```python
from build123d import *

# Parameters (mm, degrees)
EXTRUDE_2_DEPTH                = 5
SKETCH_4_W                     = 8.676470589
SKETCH_4_H                     = 35
SKETCH_4_W_2                   = 8.676470588
EXTRUDE_15_DEPTH               = 35
CUT_EXTRUDE_1_DEPTH            = 45
SKETCH_6_R                     = 14
CUT_EXTRUDE_2_DEPTH            = 45
FILLET_1_R                     = 5
SKETCH_7_R                     = 15
SKETCH_7_R_2                   = 13
EXTRUDE_16_DEPTH               = 1
SPLIT_BODIES_1_SURFACE_1_BACK  = 86
SPLIT_BODIES_1_SURFACE_1_DEPTH = 172
SPLIT_BODIES_1_SURFACE_2_BACK  = 86
SPLIT_BODIES_1_SURFACE_2_DEPTH = 172
SKETCH_17_W                    = 3
SKETCH_17_H                    = 13
EXTRUDE_20_DEPTH               = 42
EXTRUDE_21_DEPTH               = 3
SKETCH_19_R                    = 1.6
CUT_EXTRUDE_3_DEPTH            = 3
EXTRUDE_22_DEPTH               = 5
EXTRUDE_START                  = -3
EXTRUDE_25_DEPTH               = 3
HOLE_WIZARD_1_D                = 4.3
HOLE_WIZARD_1_DEPTH            = 5
HOLE_WIZARD_1_CBORE_D          = 10
HOLE_WIZARD_1_CBORE_DEPTH      = 0.5
HOLE_WIZARD_1_TIP              = 1.291850331
FILLET_2_R                     = 6


with BuildPart() as part:
    # 草图2 → 凸台-拉伸2 (new body)
    with BuildSketch(Plane.XY):
        Polygon((7.726423565, 24.338235294), (-14.773576435, 24.338235294), (-14.773576435, -35.661764706), (7.726423565, -35.661764706), (7.726423565, -23.161764706), (-6.097105846, -23.161764706), (-6.097105846, 11.838235294), (7.726423565, 11.838235294), align=None)
        Polygon((30.226423565, 24.338235294), (7.726423565, 24.338235294), (7.726423565, 11.838235294), (21.549952977, 11.838235294), (21.549952977, -23.161764706), (7.726423565, -23.161764706), (7.726423565, -35.661764706), (30.226423565, -35.661764706), align=None)
    extrude(amount=EXTRUDE_2_DEPTH)

    # 草图4 → 凸台-拉伸15 (add)
    with BuildSketch(Plane.XY.offset(5)):
        with Locations((-10.435341141, -5.661764706)):
            Rectangle(SKETCH_4_W, SKETCH_4_H)
        with Locations((25.888188271, -5.661764706)):
            Rectangle(SKETCH_4_W_2, SKETCH_4_H)
    extrude(amount=EXTRUDE_15_DEPTH)

    # 草图5 → 切除-拉伸1 (cut)
    with BuildSketch(Plane.ZY.offset(14.773576435)):
        with BuildLine():
            Line((40, -23.161764706), (40, -5.661764706))
            ThreePointArc((40, -5.661764706), (34.874368671, -18.036133377), (22.5, -23.161764706))
            Line((22.5, -23.161764706), (40, -23.161764706))
        make_face()
        with BuildLine():
            ThreePointArc((22.5, 11.838235294), (34.874368671, 6.712603965), (40, -5.661764706))
            Line((40, -5.661764706), (40, 11.838235294))
            Line((40, 11.838235294), (22.5, 11.838235294))
        make_face()
    extrude(amount=-CUT_EXTRUDE_1_DEPTH, mode=Mode.SUBTRACT)

    # 草图6 → 切除-拉伸2 (cut)
    with BuildSketch(Plane.ZY.offset(14.773576435)):
        with Locations((22.5, -5.661764706)):
            Circle(SKETCH_6_R)
    extrude(amount=-CUT_EXTRUDE_2_DEPTH, mode=Mode.SUBTRACT)

    # 圆角1
    fillet_1_edges = [part.edges().sort_by_distance(p)[0] for p in [
        (-6.097105846, 11.838235294, 2.5),
        (-6.097105846, -23.161764706, 2.5),
        (21.549952977, -23.161764706, 2.5),
        (21.549952977, 11.838235294, 2.5),
    ]]
    fillet(fillet_1_edges, radius=FILLET_1_R)

    # 草图7 → 凸台-拉伸16 (add)
    with BuildSketch(Plane(origin=(-6.097105846, 0, 0), x_dir=(0, 0, -1), z_dir=(1, 0, 0))):
        with Locations((-22.5, -5.661764706)):
            Circle(SKETCH_7_R)
        with Locations((-22.5, -5.661764706)):
            Circle(SKETCH_7_R_2, mode=Mode.SUBTRACT)
    extrude(amount=-EXTRUDE_16_DEPTH)


with BuildPart() as body_2:
    # Split Bodies 1: the piece behind the surface
    add(part.part)
    # Split Bodies 1 surface: a surface, the sketch's curves swept straight by 172 mm
    with BuildLine(Plane.XY.offset(5).offset(-SPLIT_BODIES_1_SURFACE_1_BACK), mode=Mode.PRIVATE) as split_bodies_1_surface_1_path:
        Line((7.726423565, 24.338235294), (7.726423565, -35.661764706))
    split_bodies_1_surface_1 = Shell.extrude(split_bodies_1_surface_1_path.wire(), (0 * SPLIT_BODIES_1_SURFACE_1_DEPTH, 0 * SPLIT_BODIES_1_SURFACE_1_DEPTH, 1 * SPLIT_BODIES_1_SURFACE_1_DEPTH))
    split(bisect_by=split_bodies_1_surface_1, keep=Keep.BOTTOM)


with BuildPart() as part_1:
    add(part.part)

    # Split Bodies 1: split by a surface, the side it looks to stays
    # Split Bodies 1 surface: a surface, the sketch's curves swept straight by 172 mm
    with BuildLine(Plane.XY.offset(5).offset(-SPLIT_BODIES_1_SURFACE_2_BACK), mode=Mode.PRIVATE) as split_bodies_1_surface_2_path:
        Line((7.726423565, 24.338235294), (7.726423565, -35.661764706))
    split_bodies_1_surface_2 = Shell.extrude(split_bodies_1_surface_2_path.wire(), (0 * SPLIT_BODIES_1_SURFACE_2_DEPTH, 0 * SPLIT_BODIES_1_SURFACE_2_DEPTH, 1 * SPLIT_BODIES_1_SURFACE_2_DEPTH))
    split(bisect_by=split_bodies_1_surface_2, keep=Keep.TOP)

    # 草图17 → 凸台-拉伸20 (add)
    with BuildSketch(Plane.XY.offset(5)):
        with Locations((28.726423565, -36.661764706)):
            Rectangle(SKETCH_17_W, SKETCH_17_H)
        with Locations((28.726423565, 23.338235294)):
            Rectangle(SKETCH_17_W, SKETCH_17_H)
    extrude(amount=EXTRUDE_20_DEPTH)

    # 草图18 → 凸台-拉伸21 (add)
    with BuildSketch(Plane(origin=(30.226423565, 0, 0), x_dir=(0, 0, -1), z_dir=(1, 0, 0))):
        with BuildLine():
            Line((-47, -30.161764706), (-47, -43.161764706))
            ThreePointArc((-47, -43.161764706), (-53.5, -36.661764706), (-47, -30.161764706))
        make_face()
        with BuildLine():
            Line((-47, 16.838235294), (-47, 29.838235294))
            ThreePointArc((-47, 29.838235294), (-53.5, 23.338235294), (-47, 16.838235294))
        make_face()
    extrude(amount=-EXTRUDE_21_DEPTH)

    # 草图19 → 切除-拉伸3 (cut)
    with BuildSketch(Plane(origin=(30.226423565, 0, 0), x_dir=(0, 0, -1), z_dir=(1, 0, 0))):
        with Locations((-47, 23.338235294)):
            Circle(SKETCH_19_R)
        with Locations((-47, -36.661764706)):
            Circle(SKETCH_19_R)
        with Locations((-10, 23.338235294)):
            Circle(SKETCH_19_R)
        with Locations((-10, -36.661764706)):
            Circle(SKETCH_19_R)
    extrude(amount=-CUT_EXTRUDE_3_DEPTH, mode=Mode.SUBTRACT)

    # 草图21 → 凸台-拉伸22 (add)
    with BuildSketch(Plane.XY.offset(5)):
        Polygon((18.226423565, -35.661764706), (30.226423565, -35.661764706), (30.226423565, -43.161764706), (27.226423565, -43.161764706), (26.408241747, -43.161764706), align=None)
        Polygon((18.226423565, 24.338235294), (30.226423565, 24.338235294), (30.226423565, 29.838235294), (26.476423565, 29.838235294), align=None)
    extrude(amount=-EXTRUDE_22_DEPTH)

    # 草图24 → 凸台-拉伸25 (add)
    with BuildSketch(Plane(origin=(30.226423565, 0, 0), x_dir=(0, 0, -1), z_dir=(1, 0, 0)).offset(EXTRUDE_START)):
        with BuildLine():
            Line((-5, 16.838235294), (-38, 16.838235294))
            ThreePointArc((-38, 16.838235294), (-36.230441453, 9.650254496), (-38, 2.462273699))
            ThreePointArc((-38, 2.462273699), (-31.557574949, 9.311890026), (-22.5, 11.838235294))
            Line((-22.5, 11.838235294), (-5, 11.838235294))
            Line((-5, 11.838235294), (-5, 16.838235294))
        make_face()
        with BuildLine():
            Line((-5, -30.161764706), (-38, -30.161764706))
            ThreePointArc((-38, -30.161764706), (-35.984258471, -21.973783908), (-38, -13.785803111))
            ThreePointArc((-38, -13.785803111), (-31.557574949, -20.635419438), (-22.5, -23.161764706))
            Line((-22.5, -23.161764706), (-5, -23.161764706))
            Line((-5, -23.161764706), (-5, -30.161764706))
        make_face()
    extrude(amount=EXTRUDE_25_DEPTH)

    # 打孔尺寸(%根据六角头螺)栓 全螺纹的类型1
    with Locations(Plane(origin=(18.226423565, 18.088235294, 5), x_dir=(1, 0, 0), z_dir=(0, 0, 1))):
        with Locations((0, 0), (0, -47.5)):
            CounterBoreHole(HOLE_WIZARD_1_D / 2, HOLE_WIZARD_1_CBORE_D / 2, HOLE_WIZARD_1_CBORE_DEPTH, depth=HOLE_WIZARD_1_DEPTH)
            with Locations((0, 0, -(HOLE_WIZARD_1_DEPTH + HOLE_WIZARD_1_TIP / 2))):  # 118° drill point
                Cone(0, HOLE_WIZARD_1_D / 2, HOLE_WIZARD_1_TIP, mode=Mode.SUBTRACT)

    # 圆角2
    fillet_2_edges = [part_1.edges().sort_by_distance(p)[0] for p in [
        (18.226423565, -35.661764706, 2.5),
        (18.226423565, 24.338235294, 2.5),
    ]]
    fillet(fillet_2_edges, radius=FILLET_2_R)


solid = part_1.part
```
Part model, mm, in its own coordinate system. A direction names the side the tool comes from. Coordinates: 2 decimals unless noted, no trailing zeros. Order: outer loops, then holes, each group sorted by start corner. A loop starts at its lowest first (then second) coordinate and runs counter-clockwise, first axis right, second up. Notation, with made-up numbers: (-9.75, 48.25) - (2.25, 48.25) arc R25 ccw to (2.25, 77.25) - close; hole circle Ø11 at (71.25, 42). An arc over 180 degrees is marked (long way). Return JSON: item names as keys, results as strings. Group by question number.
Item 1: Which spindle directions (+Z, -Z, +X, -X, +Y, -Y) get a long thin tool onto all of the face, cutting with end or side? Do faces 4 (the face through (24, 11.838, 14)), 5 (the face through (29, -30.162, 42)), 6 (the face through (12, -23.162, 2)), 7 (the face through (12, 24.338, 2)), 8 (the face through (27.226, -35, 29)). Say none if no direction does.
Item 2: Cut at A-A (z = 16). List the corners of the cut face in (x, y).
Item 3: Pin check, flat tips, straight feed: pin 1 (5 mm diameter, centred on x = 20, y = -29.5, fed in from +Z); pin 2 (10 mm diameter, centred on x = 16.5, z = 5.5, fed in from -Y); pin 3 (10 mm diameter, centred on x = 14, y = -26.5, fed in from +Z). Stop position of each tip, or through.
Item 4: Pull direction Z, two halves, no side cores. Call faces 1 (the face through (7.726, 18, 2)), 2 (the face through (24, -6, 0)), 3 (the face through (28.7, -38.1, 46.3)): pulls with the +Z half, pulls with the -Z half, needs draft (parallel to the pull), parting line crosses it, or undercut.
Item 5: Cut at B-B (z = 10). List the corners of the cut face in (x, y), plus the area to 3 significant figures.
Item 6: Cut at C-C (x = 28.75). List the corners of the cut face in (y, z).
Item 7: Cut at D-D (z = 30.5). List the corners of the cut face in (x, y).
Item 8: Drill centre lines: probe 1 along Y at (x, z) = (28.85, 10); probe 2 along Z at (x, y) = (23.25, 17); probe 3 along X at (y, z) = (-30, 10.5). Where is each one in solid material? Low to high. Write a range as from..to.
Check values:
{
 "1": {"face 4": "+Z, -X, +Y", "face 5": "+Z, +X, -X", "face 6": "+Z, -Z, -X", "face 7": "+Z, -Z, -X, +Y", "face 8": "+Z, -X, -Y"},
 "2": {"outline": "(21.55, -23.16) - (27.23, -23.16) - (27.23, -43.16) - (30.23, -43.16) - (30.23, -18.06) - (21.55, -18.06) - close; (21.55, 6.74) - (30.23, 6.74) - (30.23, 29.84) - (27.23, 29.84) - (27.23, 11.84) - (21.55, 11.84) - close"},
 "3": {"pin 1": "stops at z = 4.5", "pin 2": "stops at y = -38.64", "pin 3": "stops at z = 5"},
 "4": {"face 1": "needs draft", "face 2": "pulls with the -Z half", "face 3": "undercut"},
 "5": {"outline": "(21.55, -23.16) - (27.23, -23.16) - (27.23, -35.06) - (30.23, -35.06) - (30.23, -11.97) - (21.55, -11.97) - close; (21.55, 0.64) - (30.23, 0.64) - (30.23, 21.74) - (27.23, 21.74) - (27.23, 11.84) - (21.55, 11.84) - close; (27.23, -43.16) - (30.23, -43.16) - (30.23, -38.26) - (27.23, -38.26) - close; (27.23, 24.94) - (30.23, 24.94) - (30.23, 29.84) - (27.23, 29.84) - close", "area": "289 mm2"},
 "6": {"outline": "(-43.16, 0) - (29.84, 0) - (29.84, 47) arc R6.5 ccw to (16.84, 47) - (16.84, 38) arc R15.48 cw to (2.46, 38) arc R17.5 ccw to (-13.79, 38) arc R17.64 cw to (-30.16, 38) - (-30.16, 47) arc R6.5 ccw to (-43.16, 47) - close; hole circle Ø3.2 at (-36.66, 10); hole circle Ø3.2 at (-36.66, 47); hole circle Ø28 at (-5.66, 22.5); hole circle Ø3.2 at (23.34, 10); hole circle Ø3.2 at (23.34, 47)"},
 "7": {"outline": "(21.55, -21.23) - (27.23, -21.23) - (27.23, -43.16) - (30.23, -43.16) - (30.23, -17.15) - (21.55, -17.15) - close; (21.55, 5.83) - (30.23, 5.83) - (30.23, 29.84) - (27.23, 29.84) - (27.23, 9.9) - (21.55, 9.9) - close"},
 "8": {"probe 1": "y = -43.16..-38.26, -35.06..-11.97, 0.64..21.74, 24.94..29.84", "probe 2": "z = 0..5", "probe 3": "x = 27.23..30.23"}
}
